Read the model definition and answer for the solid it produces. Units are mm, in the model's axes. Face numbers are marked on the shaded views. A direction names the side the tool comes from. Round coordinates to 2 decimals unless told otherwise and drop trailing zeros. Loops run counter-clockwise (first coordinate to the right, second up) from the corner with the lowest first, then second, coordinate; pieces in that order, holes last. Notation, with made-up numbers: M 9.25,59.25 L 18.25,59.25 A17 ccw 18.25,72.25 Z; hole C -22.5,33 d1. An arc over 180 degrees is marked long. Write each question's results on one line, items separated by ' | '.
from build123d import *

# Parameters (mm, degrees)
SKETCH1_R            = 14
BOSS_EXTRUDE1_DEPTH  = 7
CHAMFER1_SIZE        = 1
SKETCH11_R           = 12
CUT_EXTRUDE3_DEPTH   = 4
M3_CLEARANCE_HOLE2_D = 3.2
SKETCH2_R            = 4
SKETCH2_R_2          = 2.5
CUT_EXTRUDE4_DEPTH   = 3
CHAMFER2_SIZE        = 0.5
CUT_EXTRUDE2_DEPTH   = 14
CIRPATTERN1_COUNT    = 4
SKETCH12_R           = 4.5
SKETCH12_R_2         = 4
BOSS_EXTRUDE3_DEPTH  = 17


with BuildPart() as part:
    # Sketch1 → Boss-Extrude1 (new body)
    with BuildSketch(Plane(origin=(0, 0, 0), x_dir=(1, 0, 0), z_dir=(0, 1, 0))):
        Circle(SKETCH1_R)
    extrude(amount=BOSS_EXTRUDE1_DEPTH)

    # Chamfer1
    chamfer1_edges = [part.edges().sort_by_distance(p)[0] for p in [
        (-14, 0, 0),
    ]]
    chamfer(chamfer1_edges, length=CHAMFER1_SIZE)

    # Sketch11 → Cut-Extrude3 (cut)
    with BuildSketch(Plane(origin=(0, 7, 0), x_dir=(1, 0, 0), z_dir=(0, 1, 0))):
        Circle(SKETCH11_R)
    extrude(amount=-CUT_EXTRUDE3_DEPTH, mode=Mode.SUBTRACT)

    # M3 Clearance Hole2 (through all)
    with Locations(Plane(origin=(0, 0, 0), x_dir=(-1, 0, 0), z_dir=(0, -1, 0))):
        with Locations((9.5, 0), (-9.5, 0), (0, 8), (0, -8)):
            Hole(M3_CLEARANCE_HOLE2_D / 2)

    # Sketch2 → Cut-Extrude4 (cut)
    with BuildSketch(Plane.XZ):
        Circle(SKETCH2_R)
        with Locations((6.01040764, 6.01040764)):
            Circle(SKETCH2_R_2)
        with Locations((6.01040764, -6.01040764)):
            Circle(SKETCH2_R_2)
        with Locations((-6.01040764, -6.01040764)):
            Circle(SKETCH2_R_2)
        with Locations((-6.01040764, 6.01040764)):
            Circle(SKETCH2_R_2)
    extrude(amount=-CUT_EXTRUDE4_DEPTH, mode=Mode.SUBTRACT)

    # Chamfer2
    chamfer2_edges = [part.edges().sort_by_distance(p)[0] for p in [
        (-4, 0, 0),
    ]]
    chamfer(chamfer2_edges, length=CHAMFER2_SIZE)

    # Sketch10 → Cut-Extrude2 (cut)
    with BuildSketch(Plane(origin=(0, 0, 0), x_dir=(0, 0, -1), z_dir=(1, 0, 0))):
        with BuildLine():
            Line((-4.5, 6), (4.5, 6))
            ThreePointArc((4.5, 6), (6, 4.5), (4.5, 3))
            Line((4.5, 3), (-4.5, 3))
            ThreePointArc((-4.5, 3), (-6, 4.5), (-4.5, 6))
        make_face()
    cut_extrude2 = extrude(amount=-CUT_EXTRUDE2_DEPTH, mode=Mode.SUBTRACT)

    # CirPattern1: Cut-Extrude2 ×4 about axis
    cirpattern1_axis = Axis((0, 3, 0), (0, 1, 0))
    for i in range(1, CIRPATTERN1_COUNT):
        add(cut_extrude2.rotate(cirpattern1_axis, i * 360 / CIRPATTERN1_COUNT), mode=Mode.SUBTRACT)

    # Sketch12 → Boss-Extrude3 (add)
    with BuildSketch(Plane(origin=(0, 3, 0), x_dir=(1, 0, 0), z_dir=(0, 1, 0))):
        Circle(SKETCH12_R)
        Circle(SKETCH12_R_2, mode=Mode.SUBTRACT)
    extrude(amount=BOSS_EXTRUDE3_DEPTH)


solid = part.part
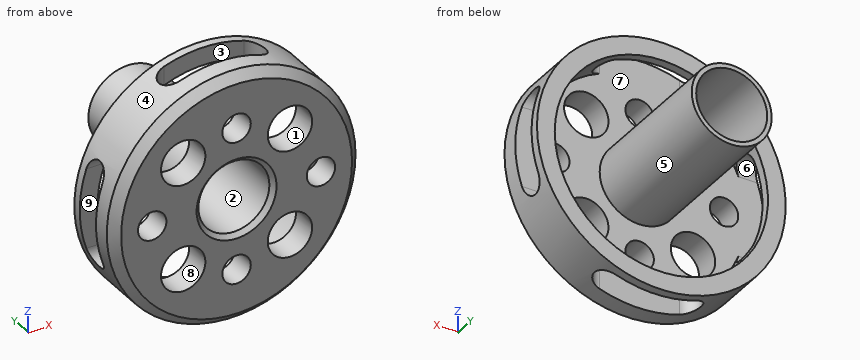
Item 1: Flat-ended cylindrical pins translate along their axes: pin 1 (6 mm diameter, centred on x = -6.01, z = -6.01, fed in from +Y); pin 2 (4 mm diameter, centred on x = 4.5, y = 13.5, fed in from -Z); pin 3 (12 mm diameter, centred on y = 10, z = 7, fed in from -X). Find the tip coordinate at first contact, or state that the pin passes through.
Outcome:
pin 1: stops at y = 3 | pin 2: stops at z = -3.74 | pin 3: stops at x = -13.88
Item 2: Straight lines are drawn through the part: line 1 (Z direction, x = 0, y = 1.8); line 2 (Y direction, x = -3.5, z = -12.25); line 3 (X direction, y = 16, z = 0). For each, find the intervals that lie inside material, in ascending order.
Outcome:
line 1: z = -14 to -9.6, -6.4 to -4, 4 to 6.4, 9.6 to 14 | line 2: y = 0 to 3, 6 to 7 | line 3: x = -4.5 to -4, 4 to 4.5
Item 3: The part is cut by section D-D (y = 12). Determine the outline of the cut face in (x, z).
Outcome:
outline: C 0,0 d9; hole C 0,0 d8
Item 4: The mould has two halves that part along Z. Classify the marked faces 1, 2, 3 and 4: pulls with the +Z half, pulls with the -Z half, needs draft (parallel to the pull), parting line crosses it, or undercut.
Outcome:
face 1: undercut | face 2: undercut | face 3: needs draft | face 4: parting line crosses it
Item 5: The part is cut by section B-B (y = 4). Determine the outline of the cut face in (x, z), plus the area to 3 significant figures.
Outcome:
outline: M -12.69,-5.91 A14 ccw -5.91,-12.69 L -5.91,-10.44 A12 cw -10.44,-5.91 Z; M -12.69,5.91 L -10.44,5.91 A12 cw -5.91,10.44 L -5.91,12.69 A14 ccw Z; C 0,0 d9; M 5.91,-12.69 A14 ccw 12.69,-5.91 L 10.44,-5.91 A12 cw 5.91,-10.44 Z; M 5.91,10.44 A12 cw 10.44,5.91 L 12.69,5.91 A14 ccw 5.91,12.69 Z; hole C 0,0 d8 | area: 78.4 mm2
Item 6: The part is cut by section A-A (z = 0). State how many separate pieces and enclosed holes the cut face has, plus the area to 4 significant figures.
Outcome:
separate pieces: 6 | enclosed holes: 0 | area: 60.55 mm2
Item 7: For the marked faces 5, 6, 7, 8 and 9, determine the directions among +Z, -Z, +X, -X, +Y, -Y from which every point of the face is accessible in a straight line to the end or side of a thin tool.
Outcome:
face 5: +Y | face 6: +X, -X | face 7: none | face 8: +Y, -Y | face 9: -X
